Autodesk Inventor part; units mm, degrees
ref_plane "YZ Plane" through (0, 0, 0) normal (1, 0, 0) x (0, 1, 0)
ref_plane "XZ Plane" through (0, 0, 0) normal (0, 1, 0) x (-1, 0, 0)
ref_plane "XY Plane" through (0, 0, 0) normal (0, 0, 1) x (1, 0, 0)
sketch "스케치1" plane through (0, 0, 0) normal (0, 0, 1) x (1, 0, 0)
  circle A0 centre (0, 0) radius 2.5
  line L0 (-6.35, 0) -> (6.35, 0) construction
  line L1 (-6.35, -1.9) -> (6.35, -1.9)
  line L2 (6.35, 1.9) -> (-6.35, 1.9)
  arc A1 (-6.35, 1.9) -> (-6.35, -1.9) centre (-6.35, 0) ccw
  arc A2 (6.35, -1.9) -> (6.35, 1.9) centre (6.35, 0) ccw
  line L3 (0, 14.5) -> (0, -14.5) construction
  circle A3 centre (0, 14.5) radius 0.5
  circle A4 centre (0, -14.5) radius 0.5
  circle A5 centre (6.35, 0) radius 0.5
  circle A6 centre (-6.35, 0) radius 0.5
  circle A7 centre (-4.25, 0) radius 0.5
  circle A8 centre (4.25, 0) radius 0.5
  line L4 (0, -1.9) -> (0, -18.5)
  line L5 (0, 1.9) -> (0, 15.9)
  arc A9 (1.9954, 14.0355) -> (-1.9954, 14.0355) centre (0, 13.9) ccw
  arc A10 (-1.9969, -16.6117) -> (1.9969, -16.6117) centre (0, -16.5) ccw
  circle A11 centre (0, 0) radius 3.4
  line L6 (-1.9954, 14.0355) -> (-2.8196, 1.9)
  line L7 (1.9954, 14.0355) -> (2.8196, 1.9)
  line L8 (-2.8196, -1.9) -> (-1.9969, -16.6117)
  line L9 (2.8196, -1.9) -> (1.9969, -16.6117)
  circle A12 centre (0, 12.5) radius 0.5
  circle A13 centre (0, 10.5) radius 0.5
  circle A14 centre (0, 8.5) radius 0.5
  circle A15 centre (0, 6.5) radius 0.5
  circle A16 centre (0, 4.5) radius 0.5
  circle A17 centre (0, 0) radius 2.35
  circle A18 centre (0, -16.5) radius 0.5
  circle A19 centre (0, -12.5) radius 0.5
  circle A20 centre (0, -10.5) radius 0.5
  circle A21 centre (0, -8.5) radius 0.5
  circle A22 centre (0, -6.5) radius 0.5
  circle A23 centre (0, -4.5) radius 0.5
  dimension "d0" = 5
  dimension "d1" = 1.9
  dimension "d2" = 16.5
  dimension "d3" = 29
  dimension "d4" = 1
  dimension "d5" = 1
  dimension "d6" = 1
  dimension "d7" = 1
  dimension "d10" = 2.1
  dimension "d17" = 2.1
  dimension "d24" = 16.6
  dimension "d25" = 14
  dimension "d26" = 4
  dimension "d27" = 4
  dimension "d28" = 6.8
  dimension "d31" = 2
  dimension "d36" = 4.7
  dimension "d39" = 2
  dimension "d46" = 2
extrude "돌출1" add sketch "스케치1" along normal blind 2.2 contours A0 L1 A17 L2 | A0 L2 A11 L1 | L2 A17 L5 A0 | A0 L5 A11 L2 | L1 A11 L4 A0 | A0 L4 A17 L1 | L5 A17 L2 A0 | A0 L2 A11 L5 | A17 L1 L2 | L2 L5 A17 | L4 A11 L1 A0 | A0 L1 A17 L4 | A17 L4 L1 | L2 A17 L1 A0 | A0 L1 A11 L2 | L5 L2 A17 | A17 L1 L4
extrude "돌출2" add sketch "스케치1" against normal blind 2.11 contours A0 L1 A17 L2 | A0 L2 A11 L1 | L2 A17 L5 A0 | A0 L5 A11 L2 | L1 A11 L4 A0 | A0 L4 A17 L1 | L5 A17 L2 A0 | A0 L2 A11 L5 | L2 A2 L1 A11 | A11 L5 A16 A15 A14 A13 A12 A3 A9 L7 | A17 L1 L2 | L2 L5 A17 | L4 A11 L1 A0 | A0 L1 A17 L4 | A17 L4 L1 | L9 A10 L4 A18 A4 A19 A20 A21 A22 A23 A11 | L2 A17 L1 A0 | A0 L1 A11 L2 | L5 L2 A17 | A11 L6 A9 L5 A3 A12 A13 A14 A15 A16 | A17 L1 L4 | L4 A23 A22 A21 A20 A19 A4 A18 A10 L8 A11 | A11 L1 A1 L2
extrude "돌출3" cut sketch "스케치1" along normal blind 3.65 contours A17 L1 L2 | L2 L5 A17 | A17 L4 L1 | L5 L2 A17 | A17 L1 L4
sketch "스케치2" plane through (0, 0, 0) normal (0, 0, 1) x (1, 0, 0)
  circle A0 centre (0, 0) radius 1.25
  dimension "d57" = 2.5
extrude "돌출4" cut sketch "스케치2" against normal blind 7.6
sketch "스케치3" plane through (0, 0, -2.11) normal (0, 0, -1) x (-1, 0, 0)
  circle A0 centre (0, 0) radius 2.25
  dimension "d60" = 4.5
extrude "돌출5" cut sketch "스케치3" against normal blind 1
sketch "스케치4" plane through (0, 0, -2.11) normal (0, 0, -1) x (-1, 0, 0)
  point P0 (0, 0)
sketch "스케치5" plane through (0, 0, -2.11) normal (0, 0, -1) x (-1, 0, 0)
  circle A0 centre (0, 0) radius 3.4
  circle A1 centre (0, 0) radius 2.25
  dimension "d63" = 4.5
  dimension "d64" = 6.8
extrude "돌출6" add sketch "스케치5" along normal blind 0.4
sketch "스케치6" plane through (0, 0, -2.11) normal (0, 0, -1) x (-1, 0, 0)
  line L0 (0.9014, 15.3127) -> (-1.0592, 15.3127)
  line L1 (-1.0592, 15.3127) -> (-1.0592, 3.6394)
  line L2 (-1.0592, 3.6394) -> (0.9014, 3.6394)
  line L3 (0.9014, 3.6394) -> (0.9014, 15.3127)
  line L4 (1.0141, -3.7747) -> (-1.0592, -3.7747)
  line L5 (-1.0592, -3.7747) -> (-1.0592, -17.386)
  line L6 (-1.0592, -17.386) -> (1.0141, -17.386)
  line L7 (1.0141, -17.386) -> (1.0141, -3.7747)
  point P0 (0, 0)
extrude "돌출7" add sketch "스케치6" against normal blind 2.11
sketch "스케치7" plane through (0, 0, -2.11) normal (0, 0, -1) x (-1, 0, 0)
  circle A0 centre (0, 14.3) radius 0.5
  arc A1 (1.9954, 14.0355) -> (-1.9954, 14.0355) centre (0, 13.9) ccw
  line L0 (0, 0) -> (0, 0.7105)
  line L1 (0, 0) -> (0.8275, 0)
  circle A2 centre (0, 12.3) radius 0.5
  circle A3 centre (0, 10.3) radius 0.5
  circle A4 centre (0, 8.3) radius 0.5
  circle A5 centre (0, 6.3) radius 0.5
  circle A6 centre (0, 4.3) radius 0.5
  line L2 (0, 15.9) -> (3.4178, 15.9)
  arc A7 (1.9954, 14.0355) -> (-1.9954, 14.0355) centre (0, 13.9) ccw
  circle A8 centre (0, -16.9) radius 0.5
  arc A9 (-1.9969, -16.6117) -> (1.9969, -16.6117) centre (0, -16.5) ccw
  circle A10 centre (0, -14.9) radius 0.5
  circle A11 centre (0, -12.9) radius 0.5
  circle A12 centre (0, -10.9) radius 0.5
  circle A13 centre (0, -8.9) radius 0.5
  circle A14 centre (0, -6.9) radius 0.5
  circle A15 centre (0, -4.9) radius 0.5
  point P0 (0, -18.5)
  dimension "d69" = 1
  dimension "d73" = 2
  dimension "d78" = 1.6
  dimension "d79" = 1
  dimension "d80" = 1.6
  dimension "d86" = 2
extrude "돌출8" cut sketch "스케치7" against normal blind 2.11
sketch "스케치9" plane through (0, 0, -2.11) normal (0, 0, -1) x (-1, 0, 0)
  circle A0 centre (0, 8.3) radius 0.5
  line L0 (0.5, 8.3) -> (3.8465, 8.3)
  line L1 (3.8465, 8.3) -> (3.8465, 17.7965)
  line L2 (3.8465, 17.7965) -> (-4.3088, 17.7965)
  line L3 (-4.3088, 17.7965) -> (-4.3088, 8.3)
  line L4 (-4.3088, 8.3) -> (0.2806, 8.3)
  circle A1 centre (0, -8.9) radius 0.5
  line L5 (0, -8.9) -> (5.2333, -8.9)
  line L6 (5.2333, -8.9) -> (5.2333, -19.7775)
  line L7 (5.2333, -19.7775) -> (-4.9031, -19.7775)
  line L8 (-4.9031, -19.7775) -> (-4.9031, -8.9)
  line L9 (-4.9031, -8.9) -> (0, -8.9)
  point P0 (0, 0)
  point P1 (0.5, -8.9)
  point P2 (-0.5, -8.9)
  point P3 (-0.5, 8.3)
extrude "돌출9" cut sketch "스케치9" against normal blind 10 contours A0 L4 L3 L2 L1 L0 | L5 L6 L7 L8 L9 A1
sketch "스케치10" plane through (0, 0, -2.11) normal (0, 0, -1) x (-1, 0, 0)
  line L0 (-0.0004, 7.8) -> (4.3151, 7.8)
  line L1 (4.3151, 7.8) -> (3.7805, 10.6296)
  line L2 (3.7805, 10.6296) -> (-3.3513, 10.6296)
  line L3 (-3.3513, 10.6296) -> (-3.4414, 7.8)
  line L4 (-3.4414, 7.8) -> (-0.0004, 7.8)
  arc A0 (-0.5, 8.3) -> (0.5, 8.3) centre (0, 8.3) ccw
  arc A1 (0.5, -8.9) -> (-0.5, -8.9) centre (0, -8.9) ccw
  line L5 (0, -8.4) -> (4.5069, -8.4)
  line L6 (4.5069, -8.4) -> (4.5069, -10.1694)
  line L7 (4.5069, -10.1694) -> (-4.0138, -10.1694)
  line L8 (-4.0138, -10.1694) -> (-4.0138, -8.4)
  line L9 (-4.0138, -8.4) -> (0, -8.4)
  point P0 (0, 0)
extrude "돌출10" cut sketch "스케치10" against normal blind 10
fillet "모깎기1" radius 2 2 edges at (-2.4189, 7.8, -1.055) (-2.4561, -8.4, -1.055)
sketch "스케치11" plane through (0, 0, -2.11) normal (0, 0, -1) x (-1, 0, 0)
  line L0 (-6.35, -1.9) -> (-2.8196, -1.9)
  line L1 (-2.8196, 1.9) -> (-6.35, 1.9)
  circle A0 centre (0, 6.3) radius 0.5
  circle A1 centre (0, -6.9) radius 0.5
  line L2 (2.8196, 1.9) -> (2.5455, 5.9355)
  line L3 (-2.5455, 5.9355) -> (-2.8196, 1.9)
  line L4 (0.5501, 7.8) -> (-0.5501, 7.8)
  line L5 (-2.8196, -1.9) -> (-2.5617, -6.5117)
  line L6 (2.5617, -6.5117) -> (2.8196, -1.9)
  point P0 (0, 0)
  point P1 (-4.5848, -1.9)
  point P2 (-4.5848, 1.9)
  point P3 (0, 7.8)
  dimension "d95" = 3.8
  dimension "d96" = 6.3
  dimension "d97" = 6.9
  dimension "d98" = 7.77
  dimension "d99" = 7.8
  dimension "d100" = 6.401
sketch "스케치12" plane through (0, 0, -2.11) normal (0, 0, -1) x (-1, 0, 0)
  line L0 (2.5785, 5.3) -> (-2.5887, 5.3)
  line L1 (-2.5455, 5.9355) -> (-2.8196, 1.9)
  circle A0 centre (0, 4.3) radius 0.5
  line L2 (3.3006, -5.9) -> (-2.5959, -5.9)
  line L3 (-2.8196, -1.9) -> (-2.5617, -6.5117)
  circle A1 centre (0, -4.9) radius 0.5
  line L4 (2.8196, 1.9) -> (6.35, 1.9)
  line L5 (5.3, 1.9) -> (5.3, -1.9)
  circle A2 centre (4.25, 0) radius 0.5
  line L6 (-6.35, 1.9) -> (-2.8196, 1.9)
  line L7 (-5.3, 1.9) -> (-5.3, -2.6397)
  circle A3 centre (-4.25, 0) radius 0.5
  line L8 (5.3, 1.9) -> (9.4862, 1.9)
  line L9 (9.4862, 1.9) -> (9.4862, -2.8158)
  line L10 (9.4862, -2.8158) -> (5.3, -2.8158)
  line L11 (5.3, -2.8158) -> (5.3, 1.9)
  line L12 (3.3006, -5.9) -> (-3.636, -5.9)
  line L13 (-3.636, -5.9) -> (-3.636, -9.5734)
  line L14 (-3.636, -9.5734) -> (3.3006, -9.5734)
  line L15 (3.3006, -9.5734) -> (3.3006, -5.9)
  line L16 (-5.3, -2.6397) -> (-8.4677, -2.6397)
  line L17 (-8.4677, -2.6397) -> (-8.4677, 1.9)
  line L18 (-8.4677, 1.9) -> (-5.3, 1.9)
  line L19 (-5.3, 1.9) -> (-5.3, -2.6397)
  line L20 (-2.5887, 5.3) -> (3.3006, 5.3)
  line L21 (3.3006, 5.3) -> (3.3006, 8.0343)
  line L22 (3.3006, 8.0343) -> (-2.5887, 8.0343)
  line L23 (-2.5887, 8.0343) -> (-2.5887, 5.3)
  point P0 (0, 0)
  point P1 (-0.0051, 5.3)
  point P2 (-2.5617, -5.9)
  point P3 (-2.5959, -5.9)
  dimension "d101" = 1
  dimension "d102" = 1
  dimension "d104" = 1.05
  dimension "d105" = 1.05
extrude "돌출11" cut sketch "스케치12" against normal blind 10 contours L7 L16 L17 L18 L6 | L0 L23 L22 L21 L20 | L15 L14 L13 L12 L2 | L4 L8 L9 L10 L11 L5
properties part number "180도 서보모터 십자축"
Design review of the part built by this model. Coordinates are the model's own, in mm. A direction names the side the tool comes from. Round coordinates to 2 decimals unless told otherwise and drop trailing zeros. Write each loop counter-clockwise with the first axis right and the second up, starting at its lowest first coordinate (ties: lowest second). Pieces come first, ordered by that corner, then holes. Notation, with made-up numbers: (-16, 23) - (-7, 23) arc R7 ccw to (-7, 33) - close; hole circle Ø11 at (-14.5, 69). An arc over 180 degrees is marked (long way). Return JSON: item names as keys, results as strings. Group by question number.
Item 1: We need section D-D on y = 4. Write out the cut boundary in (x, z), and give its area (3 significant figures).
Item 2: We need section B-B on z = -0.6. Write out the cut boundary in (x, y), and give its area (3 significant figures).
Item 3: Machinability: for faces 1 (the face through (-5.3, 0, -1)), 2 (the face through (-4, 1.9, -1)), 3 (the face through (4, -1.9, -1)), 4 (the face through (-1, -1, -1.11)), 5 (the face through (1, -1, 0)), which of the approach directions +Z, -Z, +X, -X, +Y, -Y give a long, thin tool a straight path to every point of the face, cutting with its end or side? Answer none if there is none.
Item 4: Insertion check: P1, Ø5, axis at x = 0.5, y = 1, coming from the +Z side; P2, Ø1.2, axis at x = -0.5, y = -4, coming from the +Z side; P3, Ø1, axis at x = 1, y = 4, coming from the -Z side; P4, Ø1.1, axis at x = 4, z = -1.5, coming from the +Y side. Each pin has a flat end and moves straight along its axis. Give the tip position at first contact, or say it passes through.
Item 5: For probe 1 along Y at (x, z) = (0, -1.7); probe 2 along Y at (x, z) = (0, -0.55); probe 3 along X at (y, z) = (0, 0.5), list the stretches that pass through material, from the lowest coordinate up. Write a range as [from, to].
Item 6: We need section A-A on x = 0. Give the number of separate pieces and of enclosed holes in the cut face, and give its area (3 significant figures).
Item 7: We need section C-C on x = 4.25. Write out the cut boundary in (y, z).
Model answer:
{
 "1": {"outline": "(-2.68, -2.11) - (-0.4, -2.11) - (-0.4, 0) - (-2.68, 0) - close; (0.4, -2.11) - (2.68, -2.11) - (2.68, 0) - (0.4, 0) - close", "area": "9.61 mm²"},
 "2": {"outline": "(-5.3, -1.9) - (-2.82, -1.9) - (-2.6, -5.9) - (2.6, -5.9) - (2.82, -1.9) - (5.3, -1.9) - (5.3, 1.9) - (2.82, 1.9) - (2.59, 5.3) - (-2.59, 5.3) - (-2.82, 1.9) - (-5.3, 1.9) - close; hole circle Ø1 at (-4.25, 0); hole circle Ø2.5 at (0, 0); hole circle Ø1 at (0, -4.9); hole circle Ø1 at (0, 4.3); hole circle Ø1 at (4.25, 0)", "area": "72.3 mm²"},
 "3": {"face 1": "+Z, -Z, -X, +Y, -Y", "face 2": "+Z, -Z, -X, +Y", "face 3": "+Z, -Z, +X, -Y", "face 4": "-Z", "face 5": "+Z"},
 "4": {"P1": "stops at z = 2.2", "P2": "stops at z = 0", "P3": "stops at z = -2.11", "P4": "stops at y = 1.9"},
 "5": {"probe 1": "y = [-5.9, -5.4], [-4.4, -2.25], [2.25, 3.8], [4.8, 5.3]", "probe 2": "y = [-5.9, -5.4], [-4.4, -1.25], [1.25, 3.8], [4.8, 5.3]", "probe 3": "x = [-3.4, -2.35], [2.35, 3.4]"},
 "6": {"separate pieces": "4", "enclosed holes": "0", "area": "17.7 mm²"},
 "7": {"outline": "(-1.9, -2.11) - (-0.5, -2.11) - (-0.5, 0) - (-1.9, 0) - close; (0.5, -2.11) - (1.9, -2.11) - (1.9, 0) - (0.5, 0) - close"}
}
